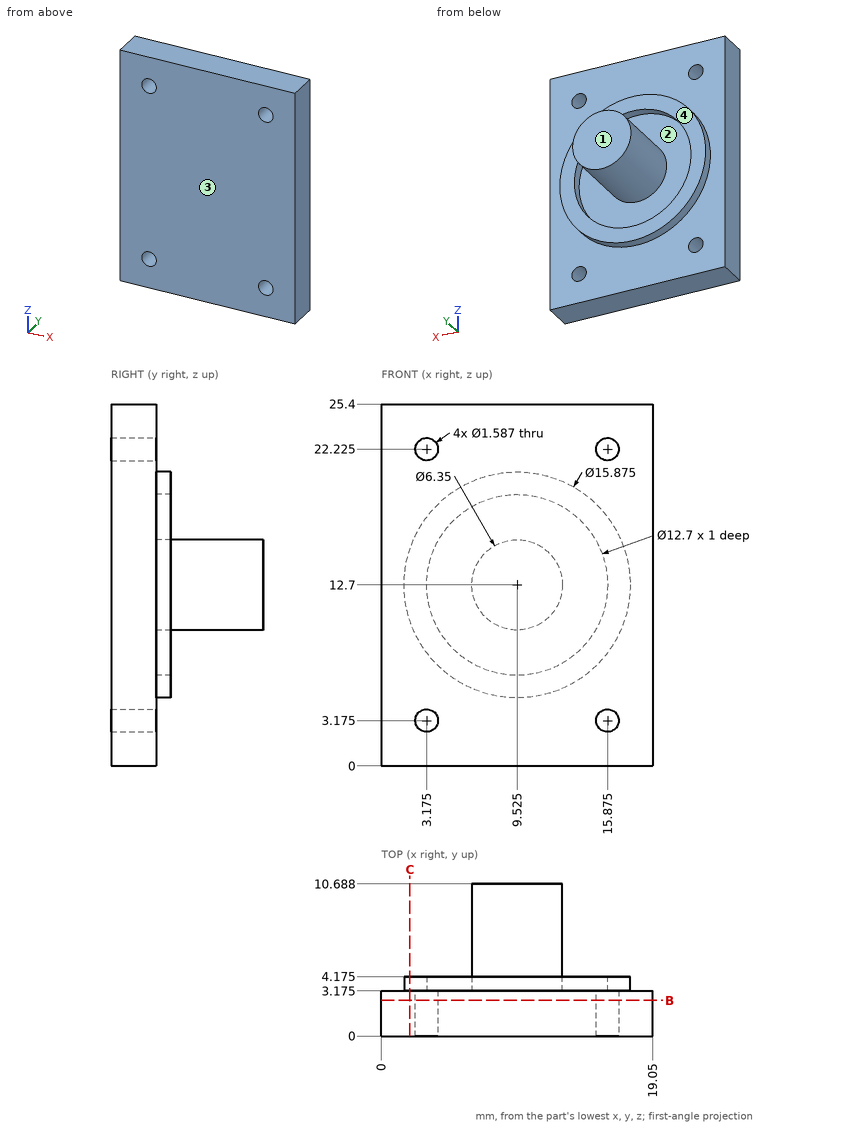
Geometry check sheet. Reference: drawing and pictorial views, mm from the part's lowest x, y, z. A direction names the side the tool comes from. Coordinates: 2 decimals unless noted, no trailing zeros. Loops run counter-clockwise (first coordinate to the right, second up) from the corner with the lowest first, then second, coordinate; pieces in that order, holes last. Notation, with made-up numbers: (-26, 89) -> (33, 89) arc R25 ccw to (33, 123) -> close; hole circle Ø6 at (44, -15.75). An arc over 180 degrees is marked (long way). Put each result on its own line as item: value.
1) Release check for a two-part mould opening along X. For the marked faces 1 and 2 record: released by +X, released by -X, zero draft, split by the parting line, or undercut.
Result set:
face 1: zero draft
face 2: undercut
2) Cross-section at B-B on y = 2.5. Count the separate pieces of the cut face and the enclosed holes in it, plus the area to 3 significant figures.
Result set:
separate pieces: 1
enclosed holes: 4
area: 476 mm^2
3) Gauge pin test, flat ends, axial feed: pin 1 Ø1.8 at (x, z) = (15.875, 3.175) entering from -Y; pin 2 Ø1.5 at (x, y) = (8.5, 6.5) entering from +Z; pin 3 Ø1.5 at (x, y) = (13, 5.5) entering from -Z; pin 4 Ø2.5 at (x, z) = (3.175, 3.175) entering from +Y (1 decimal). Record the tip position at first contact, or that the pin passes through.
Result set:
pin 1: stops at y = 0
pin 2: stops at z = 15.86
pin 3: stops at z = 11.07
pin 4: stops at y = 3.2
4) Thickness scan on line 1 (X direction, y = 3.5, z = 15.25) (1 decimal); line 2 (Y direction, x = 13.5, z = 3) (1 decimal); line 3 (Y direction, x = 15.5, z = 16.5) (1 decimal). Record the ranges inside material, lowest first.
Result set:
line 1: x = 2 to 3.7, 7.6 to 11.4, 15.3 to 17
line 2: y = 0 to 3.2
line 3: y = 0 to 4.2
5) Cross-section at C-C on x = 2. Record the boundary of the cut face in (y, z) (1 decimal).
Result set:
outline: (0, 0) -> (3.2, 0) -> (3.2, 10.2) -> (4.2, 10.2) -> (4.2, 15.2) -> (3.2, 15.2) -> (3.2, 25.4) -> (0, 25.4) -> close
6) Tool access check on the marked faces 3 and 4. Record the directions out of +Z, -Z, +X, -X, +Y, -Y that give a thin tool (end or side, any length) a straight path to the whole face; none if there is none.
Result set:
face 3: +Z, -Z, +X, -X, -Y
face 4: +Y
